from build123d import *

# Parameters (mm, degrees)
SKETCH1_R      = 2.1844
SKETCH1_R_2    = 1.1938
SKETCH1_R_3    = 4.0005
EXTRUDE1_DEPTH = 1.524
EXTRUDE3_START = -13.3731
SKETCH3_W      = 7.9502
SKETCH3_H      = 24.2062
SKETCH3_R      = 2.1844
EXTRUDE3_DEPTH = 1.524
EXTRUDE4_START = 15.8369
SKETCH3_3_W    = 41.2496
SKETCH3_3_H    = 24.2062
SKETCH3_3_R    = 1.5875
EXTRUDE4_DEPTH = 1.524
FILLET4_R      = 1.778
FILLET5_R      = 0.254


with BuildPart() as part:
    # Sketch1 → Extrude1 (new body)
    with BuildSketch(Plane(origin=(0, 0, 0), x_dir=(1, 0, 0), z_dir=(0, 1, 0))):
        Polygon((28.575, -12.4079), (28.575, 13.3731), (20.6248, 13.3731), (20.6248, 8.4201), (17.4498, 8.4201), (17.4498, 17.3609), (-17.4498, 17.3609), (-17.4498, 8.4201), (-20.6248, 8.4201), (-20.6248, 13.3731), (-28.575, 13.3731), (-28.575, -12.4079), (-20.6248, -12.4079), (-20.6248, -17.3609), (20.6248, -17.3609), (20.6248, -12.4079), align=None)
        with Locations((-24.8158, -4.3815)):
            Circle(SKETCH1_R, mode=Mode.SUBTRACT)
        with Locations((-8.3312, -2.9083)):
            Circle(SKETCH1_R_2, mode=Mode.SUBTRACT)
        with Locations((8.3312, -2.9083)):
            Circle(SKETCH1_R_2, mode=Mode.SUBTRACT)
        with Locations((24.8158, -4.3815)):
            Circle(SKETCH1_R, mode=Mode.SUBTRACT)
        with Locations((8.3312, 13.7541)):
            Circle(SKETCH1_R_2, mode=Mode.SUBTRACT)
        with Locations((-24.8158, 5.4229)):
            Circle(SKETCH1_R, mode=Mode.SUBTRACT)
        with Locations((-16.6624, 5.4229)):
            Circle(SKETCH1_R_2, mode=Mode.SUBTRACT)
        with Locations((-8.3312, 5.4229)):
            Circle(SKETCH1_R_3, mode=Mode.SUBTRACT)
        with Locations((-8.3312, 13.7541)):
            Circle(SKETCH1_R_2, mode=Mode.SUBTRACT)
        with Locations((0, 5.4229)):
            Circle(SKETCH1_R_2, mode=Mode.SUBTRACT)
        with Locations((8.3312, 5.4229)):
            Circle(SKETCH1_R_3, mode=Mode.SUBTRACT)
        with Locations((16.6624, 5.4229)):
            Circle(SKETCH1_R_2, mode=Mode.SUBTRACT)
        with Locations((24.8158, 5.4229)):
            Circle(SKETCH1_R, mode=Mode.SUBTRACT)
    extrude(amount=EXTRUDE1_DEPTH)

    # Sketch3 → Extrude3 (add)
    with BuildSketch(Plane.XY.offset(EXTRUDE3_START)):
        with Locations((-24.5999, 12.1031)):
            Rectangle(SKETCH3_W, SKETCH3_H)
        with Locations((-24.5999, 19.1262)):
            Circle(SKETCH3_R, mode=Mode.SUBTRACT)
        with Locations((-24.5999, 9.3218)):
            Circle(SKETCH3_R, mode=Mode.SUBTRACT)
        with Locations((24.5999, 12.1031)):
            Rectangle(SKETCH3_W, SKETCH3_H)
        with Locations((24.5999, 9.3218)):
            Circle(SKETCH3_R, mode=Mode.SUBTRACT)
        with Locations((24.5999, 19.1262)):
            Circle(SKETCH3_R, mode=Mode.SUBTRACT)
    extrude(amount=EXTRUDE3_DEPTH)

    # Sketch3_3 → Extrude4 (add)
    with BuildSketch(Plane.XY.offset(EXTRUDE4_START)):
        with Locations((0, 12.1031)):
            Rectangle(SKETCH3_3_W, SKETCH3_3_H)
        with Locations((-9.9314, 14.2748)):
            Circle(SKETCH3_3_R, mode=Mode.SUBTRACT)
        with Locations((9.9314, 14.2748)):
            Circle(SKETCH3_3_R, mode=Mode.SUBTRACT)
    extrude(amount=EXTRUDE4_DEPTH)

    # Fillet4
    fillet4_edges = [part.edges().sort_by_distance(p)[0] for p in [
        (0, 0, 17.3609),
        (-24.5999, 0, -13.3731),
        (24.5999, 0, -13.3731),
    ]]
    fillet(fillet4_edges, radius=FILLET4_R)

    # Fillet5
    fillet5_edges = [part.edges().sort_by_distance(p)[0] for p in [
        (24.5999, 1.524, -11.8491),
        (0, 1.524, 15.8369),
        (-24.5999, 1.524, -11.8491),
    ]]
    fillet(fillet5_edges, radius=FILLET5_R)


solid = part.part
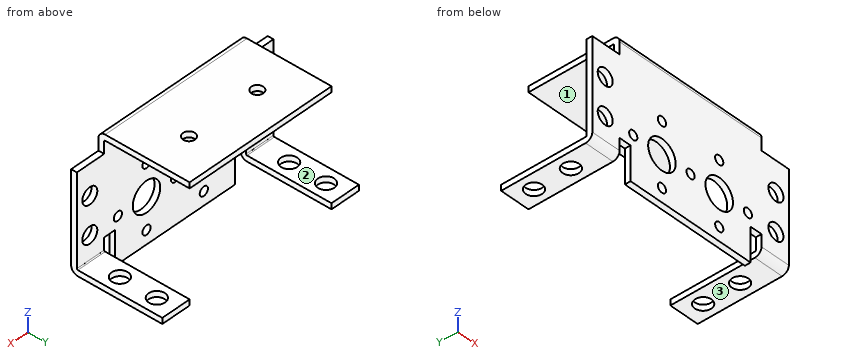
Can you work these out from the model? Positions are in its coordinate system, mm. Face numbers are marked on the shaded views. A direction names the side the tool comes from. Coordinates: 2 decimals unless noted, no trailing zeros. Order: outer loops, then holes, each group sorted by start corner. A loop starts at its lowest first (then second) coordinate and runs counter-clockwise, first axis right, second up. Notation, with made-up numbers: M 62.5,85.5 L 67.5,85.5 A34 ccw 67.5,115.5 Z; hole C 85,66.5 d2. An arc over 180 degrees is marked long. Answer as CSV lines item,"result".
(1) Suppose I cut it at D-D on z = 14.5. Please give me the cut outline in (x, y), plus the area to 3 significant figures.
Geometry check:
outline,"M -20.62,0 L 20.62,0 L 20.62,1.52 L -20.62,1.52 Z"
area,"62.9 mm^2"
(2) Suppose I cut it at B-B on x = 0. Please give me the cut outline in (y, z).
Geometry check:
outline,"M 0,-17.36 L 1.52,-17.36 L 1.52,-6.62 L 0,-6.62 Z; M 0,-4.23 L 1.52,-4.23 L 1.52,15.58 A0.25 cw 1.78,15.84 L 24.21,15.84 L 24.21,17.36 L 1.78,17.36 A1.78 ccw 0,15.58 Z"
(3) Suppose I cut it at C-C on z = 9. Please give me the cut outline in (x, y) (3 decimals), plus the area to 3 significant figures.
Geometry check:
outline,"M -28.575,0 L 28.575,0 L 28.575,1.524 L -28.575,1.524 Z"
area,"87.1 mm^2"
(4) Please list where these lines run through material, in increasing order: L1, parallel to Z at x = -20.5, y = 10.5; L2, parallel to Y at x = 20.5, z = -1; L3, parallel to Z at x = 0, y = 0.8.
Geometry check:
L1,"15.84 to 17.36"
L2,"0 to 1.52"
L3,"-17.36 to -6.62, -4.23 to 17.07"
(5) Suppose I cut it at A-A on z = -10.5. Please give me the cut outline in (x, y) (3 decimals).
Geometry check:
outline,"M -28.575,0 L -20.625,0 L -20.625,1.524 L -28.575,1.524 Z; M -17.45,0 L 17.45,0 L 17.45,1.524 L -17.45,1.524 Z; M 20.625,0 L 28.575,0 L 28.575,1.524 L 20.625,1.524 Z"
(6) I'm going to push flat-ended pins straight in: pin 1 (5 mm diameter, centred on x = -11.5, z = -7.5, fed in from +Y); pin 2 (5 mm diameter, centred on x = -24.6, y = 9.32, fed in from -Z); pin 3 (1.2 mm diameter, centred on x = 19, y = 1, fed in from -Z). Where does each tip first touch, or does it pass through?
Geometry check:
pin 1,"y = 1.52"
pin 2,"z = -13.37"
pin 3,"z = -8.42"
(7) On a 3-axis mill with a long thin cutter (end or side, diameter ignored), from which of +Z, -Z, +X, -X, +Y, -Y can I reach the whole of each face in a straight line? I mean the marked faces 1, 2 and 3. Say none if no direction works.
Geometry check:
face 1,"-Z, +X, -X, +Y"
face 2,"+Z, +X, -X, +Y"
face 3,"-Z, +X, -X, +Y, -Y"
